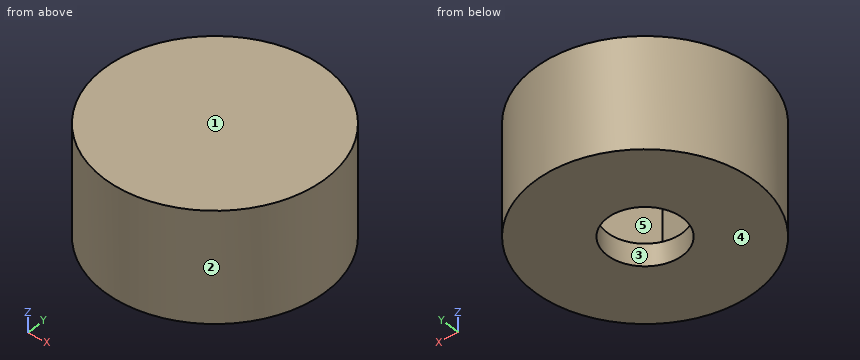
```python
from build123d import *

# Parameters (mm, degrees)
CYLINDER_R      = 10
CYLINDER_DEPTH  = 8
POCKET_DEPTH    = 6
SKETCH001_R     = 10
PAD_DEPTH       = 2
SKETCH002_R     = 3.4
POCKET001_DEPTH = 2


with BuildPart() as part:
    # Cylinder → Cylinder (new body)
    with BuildSketch(Plane.XY):
        Circle(CYLINDER_R)
    extrude(amount=CYLINDER_DEPTH)

    # Sketch (on Face2 of BaseFeature) → Pocket (cut)
    with BuildSketch(Plane.XY.offset(8)):
        Polygon((3.32, -5.750409), (6.64, 0), (3.32, 5.750409), (-3.32, 5.750409), (-6.64, 0), (-3.32, -5.750409), align=None)
    extrude(amount=-POCKET_DEPTH, mode=Mode.SUBTRACT)

    # Sketch001 (on Face2 of Pocket) → Pad (join)
    with BuildSketch(Plane.XY.offset(8)):
        Circle(SKETCH001_R)
    extrude(amount=PAD_DEPTH)

    # Sketch002 (on Face3 of Pad) → Pocket001 (cut)
    with BuildSketch(Plane(origin=(0, 0, 0), x_dir=(1, 0, 0), z_dir=(0, 0, -1))):
        Circle(SKETCH002_R)
    extrude(amount=-POCKET001_DEPTH, mode=Mode.SUBTRACT)


solid = part.part
```
Part model, mm, in its own coordinate system. Face numbers are marked on the shaded views. A direction names the side the tool comes from. Round coordinates to 2 decimals unless told otherwise and drop trailing zeros. Order: outer loops, then holes, each group sorted by start corner. A loop starts at its lowest first (then second) coordinate and runs counter-clockwise, first axis right, second up. Notation, with made-up numbers: M -22,87 L 32,87 A8 cw 32,98 Z; hole C 18.25,-6 d1. An arc over 180 degrees is marked long. Put each result on its own line as item: value. Start each with the question number.
1. Slice it at C-C on y = 4.5. List the corners of the cut face in (x, z).
2. Tool access for the marked faces 4 and 5: list every direction of +Z, -Z, +X, -X, +Y, -Y with a clear straight run to the whole face (end or side of a thin tool).
3. Slice it at A-A on z = 7.25. List the corners of the cut face in (x, y), then the cut area to 3 significant figures.
4. Drop flat-ended pins along their axis: pin 1 (4 mm diameter, centred on y = -2, z = 4.5, fed in from +X); pin 2 (3 mm diameter, centred on x = 3.5, z = 3.5, fed in from -Y); pin 3 (2 mm diameter, centred on y = 8, z = 2.5, fed in from +X); pin 4 (1 mm diameter, centred on y = 8, z = 3.5, fed in from -X). Give the stop position or say it passes through.
5. Two-plate mould, pull along Y, no slides. Class the marked faces 1, 2 and 3: +Y half, -Y half, draft (parallel to the pull), parting line (faces both ways), or undercut.
6. Slice it at D-D on x = 0. List the corners of the cut face in (y, z).
7. Slice it at B-B on x = 4.25. List the corners of the cut face in (y, z).
8. Drill centre lines: probe 1 along Y at (x, z) = (0, 1.35); probe 2 along Z at (x, y) = (-5, -0.5); probe 3 along X at (y, z) = (2.5, 5.5). Where is each one in solid material? Low to high. Write a range as [from, to].
Findings:
1. outline: M -8.93,0 L 8.93,0 L 8.93,10 L -8.93,10 Z; hole M -4.04,2 L 4.04,2 L 4.04,8 L -4.04,8 Z
2. face 4: -Z, +X, -X, +Y, -Y
2. face 5: none
3. outline: C 0,0 d20; hole M -6.64,0 L -3.32,-5.75 L 3.32,-5.75 L 6.64,0 L 3.32,5.75 L -3.32,5.75 Z
3. area: 200 mm2
4. pin 1: x = 10
4. pin 2: y = -9.8
4. pin 3: x = 7.14
4. pin 4: x = -6.61
5. face 1: draft
5. face 2: parting line
5. face 3: undercut
6. outline: M -10,0 L -3.4,0 L -3.4,2 L -5.75,2 L -5.75,8 L 5.75,8 L 5.75,2 L 3.4,2 L 3.4,0 L 10,0 L 10,10 L -10,10 Z
7. outline: M -9.05,0 L 9.05,0 L 9.05,10 L -9.05,10 Z; hole M -4.14,2 L 4.14,2 L 4.14,8 L -4.14,8 Z
8. probe 1: [-10, -3.4], [3.4, 10]
8. probe 2: [0, 2], [8, 10]
8. probe 3: [-9.68, -5.2], [5.2, 9.68]
